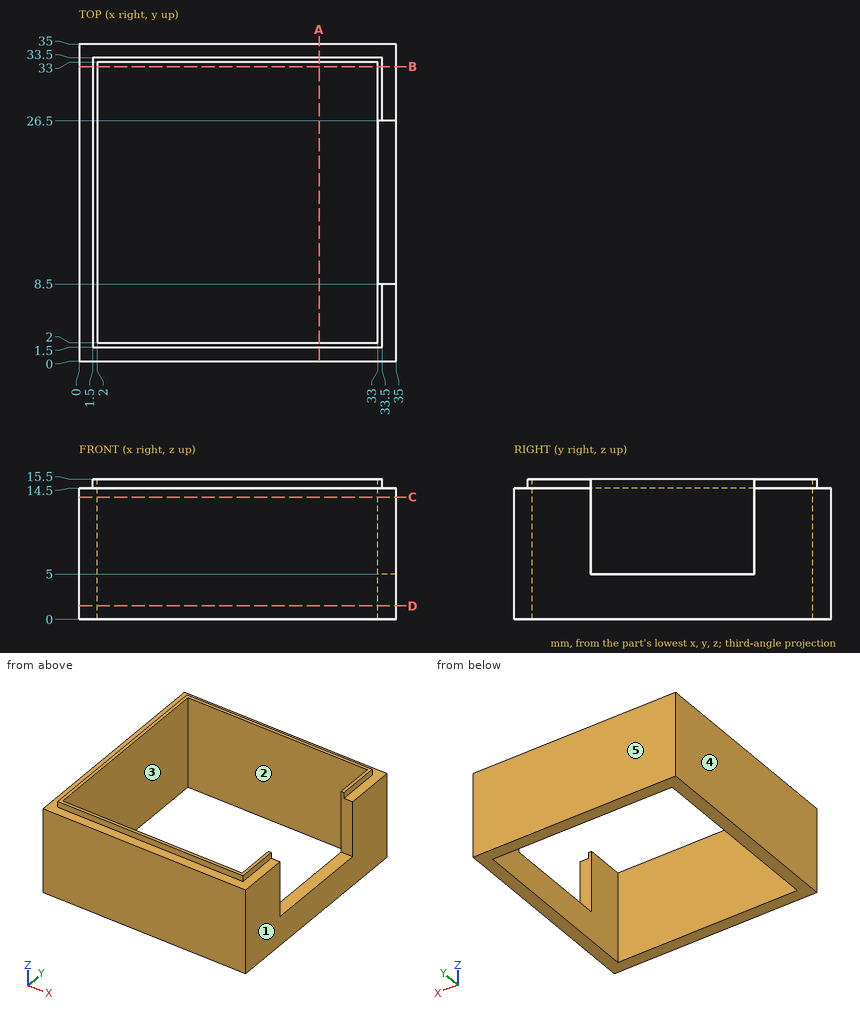
Geometry: see drawing. Coordinates: mm, zero at the bounding-box minimum. A direction names the side the tool comes from. Round coordinates to 2 decimals unless told otherwise and drop trailing zeros. Write each loop counter-clockwise with the first axis right and the second up, starting at its lowest first coordinate (ties: lowest second). Pieces come first, ordered by that corner, then holes. Notation, with made-up numbers: M 84,52.5 L 119,52.5 A13 ccw 119,76.5 Z; hole C -36,88.5 d3. An arc over 180 degrees is marked long. Answer as a JSON object with one key per item and string values. Group by question number.
(1) First-contact query: pin 1 (2 mm diameter, centred on x = 34.5, y = 20, fed in from +Z); pin 2 (0.8 mm diameter, centred on x = 22.5, z = 15, fed in from -Y); pin 3 (10.5 mm diameter, centred on x = 25, y = 23, fed in from +Z); pin 4 (0.8 mm diameter, centred on y = 29.5, z = 15, fed in from +X). Flat tips, straight axial feed; report the tip coordinate or a pass-through.
(2) Section query C-C on z = 13.5. Output: boundary loops of the cut face in (x, y), then the cut area to 3 significant figures.
(3) Reachability of the marked faces 1 and 2 from +Z, -Z, +X, -X, +Y, -Y: full face, straight path, thin tool, end or side. Return the list, or none.
(4) Ray query, line 1 (Y direction, x = 4, z = 1.5); line 2 (X direction, y = 22.5, z = 13.25). Return the intervals inside material, ascending. Write a range as [from, to].
(5) Section query A-A on x = 26.5. Output: boundary loops of the cut face in (y, z), then the cut area to 3 significant figures.
(6) Mould query, pull axis Y, two halves, no side actions, for the marked faces 3, 4 and 5. Classes: +Y half, -Y half, draft (parallel to the pull), parting line (faces both ways), or undercut.
(7) Section query D-D on z = 1.5. Output: boundary loops of the cut face in (x, y), then the cut area to 3 significant figures.
Computed values:
{
 "1": {"pin 1": "z = 5", "pin 2": "y = 1.5", "pin 3": "through", "pin 4": "x = 33.5"},
 "2": {"outline": "M 0,0 L 35,0 L 35,8.5 L 33,8.5 L 33,2 L 2,2 L 2,33 L 33,33 L 33,26.5 L 35,26.5 L 35,35 L 0,35 Z", "area": "228 mm^2"},
 "3": {"face 1": "+Z, -Z, +X, +Y, -Y", "face 2": "+Z, -Z"},
 "4": {"line 1": "[0, 2], [33, 35]", "line 2": "[0, 2]"},
 "5": {"outline": "M 0,0 L 2,0 L 2,15.5 L 1.5,15.5 L 1.5,14.5 L 0,14.5 Z; M 33,0 L 35,0 L 35,14.5 L 33.5,14.5 L 33.5,15.5 L 33,15.5 Z", "area": "59.0 mm^2"},
 "6": {"face 3": "undercut", "face 4": "draft", "face 5": "+Y half"},
 "7": {"outline": "M 0,0 L 35,0 L 35,35 L 0,35 Z; hole M 2,2 L 33,2 L 33,33 L 2,33 Z", "area": "264 mm^2"}
}
